Part print with two shaded views. Sizes in mm from the minimum x, y, z corner. A direction names the side the tool comes from. Round coordinates to 2 decimals unless told otherwise and drop trailing zeros. Loops run counter-clockwise (first coordinate to the right, second up) from the corner with the lowest first, then second, coordinate; pieces in that order, holes last. Notation, with made-up numbers: (89.25, -40) -> (146.25, -40) arc R19 cw to (146.25, -8) -> close; hole circle Ø4 at (79.5, 41). An arc over 180 degrees is marked (long way). Use a Markdown table: item, result. Add a question column.
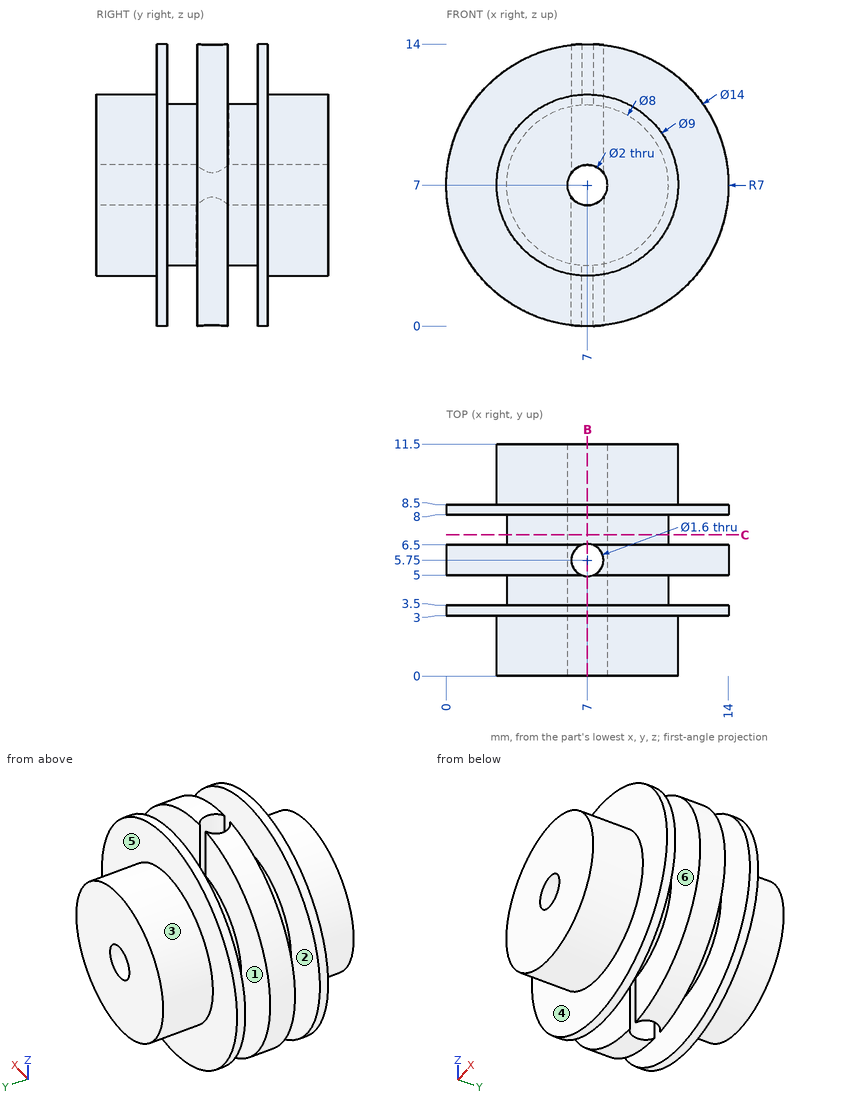
1) Tool access for the marked faces 1, 2 and 3: list every direction of +Z, -Z, +X, -X, +Y, -Y with a clear straight run to the whole face (end or side of a thin tool).
2) Cut at C-C on y = 7. Write the cut outline in (x, z), and give its area (3 significant figures).
3) Pull direction Y, two halves, no side cores. Call the marked faces 4, 5 and 6: +Y half, -Y half, draft (parallel to the pull), parting line (faces both ways), or undercut.
4) Pin check, flat tips, straight feed: pin 1 Ø2.5 at (x, y) = (7, 5.75) entering from -Z; pin 2 Ø5 at (y, z) = (8, 5) entering from +X; pin 3 Ø2 at (x, y) = (5, 6.5) entering from +Z; pin 4 Ø2.5 at (x, y) = (7, 5.75) entering from +Z. Stop position of each tip, or through.
5) Wall check: probe 1 along Y at (x, z) = (8, 13); probe 2 along Y at (x, z) = (7, 4.25); probe 3 along X at (y, z) = (6, 2). Give the ranges that are in metal, low to high. Write a range as from..to.
6) Cut at B-B on x = 7. Count the separate pieces of the cut face and the enclosed holes in it, and give its area (3 significant figures).
Established:
| question | item | result |
|---|---|---|
| 1 | face 1 | -X |
| 1 | face 2 | none |
| 1 | face 3 | +Y |
| 2 | outline | circle Ø8 at (7, 7); hole circle Ø2 at (7, 7) |
| 2 | area | 47.1 mm^2 |
| 3 | face 4 | -Y half |
| 3 | face 5 | +Y half |
| 3 | face 6 | undercut |
| 4 | pin 1 | stops at z = 0.01 |
| 4 | pin 2 | stops at x = 14 |
| 4 | pin 3 | stops at z = 13.93 |
| 4 | pin 4 | stops at z = 13.99 |
| 5 | probe 1 | y = 3..3.5, 5..6.5, 8..8.5 |
| 5 | probe 2 | y = 0..4.95, 6.55..11.5 |
| 5 | probe 3 | x = 2.1..6.24, 7.76..11.9 |
| 6 | separate pieces | 4 |
| 6 | enclosed holes | 0 |
| 6 | area | 71.4 mm^2 |
